Could you check a few things on this model? Use its own coordinates, in mm. A direction names the side the tool comes from. Coordinates: 2 decimals unless noted, no trailing zeros. Order: outer loops, then holes, each group sorted by start corner. A loop starts at its lowest first (then second) coordinate and runs counter-clockwise, first axis right, second up. Notation, with made-up numbers: M -7,-38 L 13,-38 A21 ccw 13,-1 Z; hole C 4,-35 d3. An arc over 180 degrees is marked long. Put each result on its own line as item: value. Start each with the question number.
```python
from build123d import *

# Parameters (mm, degrees)
SKETCH_1_R          = 1.5
EXTRUDE_1_DEPTH     = 4.5
FILLET_1_R          = 2
SKETCH_2_R          = 3.75
CUT_EXTRUDE_1_DEPTH = 3


with BuildPart() as part:
    # ｽｹｯﾁ1 → ﾎﾞｽ - 押し出し1 (new body)
    with BuildSketch(Plane(origin=(0, 0, 0), x_dir=(1, 0, 0), z_dir=(0, 1, 0))):
        with BuildLine():
            Line((56.137020409, 12.445277801), (68.340720498, 15.150772976))
            ThreePointArc((68.340720498, 15.150772976), (70, 0), (68.340720498, -15.150772976))
            Line((68.340720498, -15.150772976), (56.137020409, -12.445277801))
            ThreePointArc((56.137020409, -12.445277801), (57.5, 0), (56.137020409, 12.445277801))
        make_face()
        with Locations(Location((64.443915989, 8.484202494, 0), (0, 0, 270))):
            Circle(SKETCH_1_R, mode=Mode.SUBTRACT)
        with Locations(Location((64.443915989, -8.484202494, 0), (0, 0, 90))):
            Circle(SKETCH_1_R, mode=Mode.SUBTRACT)
    extrude(amount=EXTRUDE_1_DEPTH)

    # ﾌｨﾚｯﾄ1
    fillet_1_edges = [part.edges().sort_by_distance(p)[0] for p in [
        (68.340720498, 2.25, 15.150772976),
        (56.137020409, 2.25, 12.445277801),
        (56.137020409, 2.25, -12.445277801),
        (68.340720498, 2.25, -15.150772976),
    ]]
    fillet(fillet_1_edges, radius=FILLET_1_R)

    # ｽｹｯﾁ2 → ｶｯﾄ - 押し出し1 (cut)
    with BuildSketch(Plane(origin=(0, 4.5, 0), x_dir=(1, 0, 0), z_dir=(0, 1, 0))):
        with Locations(Location((64.443915989, 8.484202494, 0), (0, 0, 270))):
            Circle(SKETCH_2_R)
        with Locations(Location((64.443915989, -8.484202494, 0), (0, 0, 270))):
            Circle(SKETCH_2_R)
    extrude(amount=-CUT_EXTRUDE_1_DEPTH, mode=Mode.SUBTRACT)


solid = part.part
```
Item 1: I need wall thicknesses on probe 1 along Z at (x, y) = (65.5, 3.5); probe 2 along Z at (x, y) = (66.5, 4.25); probe 3 along Z at (x, y) = (59.25, 1.8). Which ranges of each line are inside material? Lowest first, please.
Item 2: If we section it at C-C on z = 10.25: Write out the boundary of the cut face in (x, y).
Item 3: For faces 4 (the cylindrical face through (68.162, 3.021, -8.972)), 5 (the cylindrical face through (57.5, 2.2, 0.1)), which set-ups out of +Z, -Z, +X, -X, +Y, -Y let a thin tool reach every point of the face, with its end or its side?
Item 4: If we section it at D-D on x = 61: Write out the boundary of the cut face in (y, z), then the cut area to 3 significant figures.
Item 5: If we section it at A-A on y = 0.5: Write out the boundary of the cut face in (x, z), then the cut area to 3 significant figures.
Item 6: If we section it at B-B on x = 65.5: Write out the boundary of the cut face in (y, z).
Item 7: If we mould it in two halves opening along Z, with no side actions, what happens to faces 1 (the cylindrical face through (65.775, 0.74, 7.792)), 2 (the cylindrical face through (67.91, 2.282, 14.417)), 3 (the flat face through (63, 4.5, 0))? For each: released by +Z, released by -Z, zero draft, split by the parting line, or undercut.
Item 8: For pin 1 Ø2 at (x, z) = (65, 7) entering from +Y; pin 2 Ø1 at (y, z) = (3.5, -11) entering from +X; pin 3 Ø1 at (x, y) = (61, 2.5) entering from -Z, each with a flat end and sliding along its axis, tell me the tip position at first contact or that it passes through.
Geometry check:
1. probe 1: z = -14.52 to -12.08, -4.89 to 4.89, 12.08 to 14.52
1. probe 2: z = -14.74 to -11.62, -5.35 to 5.35, 11.62 to 14.74
1. probe 3: z = -13.14 to 13.14
2. outline: M 56.58,0 L 69.25,0 L 69.25,4.5 L 67.75,4.5 L 67.75,1.5 L 61.14,1.5 L 61.14,4.5 L 56.58,4.5 Z
3. face 4: +Y
3. face 5: -X, +Y, -Y
4. outline: M 0,-13.52 L 4.5,-13.52 L 4.5,-9.97 L 1.5,-9.97 L 1.5,-7 L 4.5,-7 L 4.5,7 L 1.5,7 L 1.5,9.97 L 4.5,9.97 L 4.5,13.52 L 0,13.52 Z
4. area: 104 mm²
5. outline: M 56.52,-10.55 A2 ccw 58.06,-12.87 L 66.36,-14.71 A2 ccw 68.76,-13.13 A70 ccw 68.76,13.13 A2 ccw 66.36,14.71 L 58.06,12.87 A2 ccw 56.52,10.55 A57.5 cw Z; hole C 64.44,-8.48 d3; hole C 64.44,8.48 d3
5. area: 330 mm²
6. outline: M 0,-14.52 L 4.5,-14.52 L 4.5,-12.08 L 1.5,-12.08 L 1.5,-9.55 L 0,-9.55 Z; M 0,-7.42 L 1.5,-7.42 L 1.5,-4.89 L 4.5,-4.89 L 4.5,4.89 L 1.5,4.89 L 1.5,7.42 L 0,7.42 Z; M 0,9.55 L 1.5,9.55 L 1.5,12.08 L 4.5,12.08 L 4.5,14.52 L 0,14.52 Z
7. face 1: undercut
7. face 2: released by +Z
7. face 3: zero draft
8. pin 1: stops at y = 1.5
8. pin 2: stops at x = 69.21
8. pin 3: stops at z = -13.63
